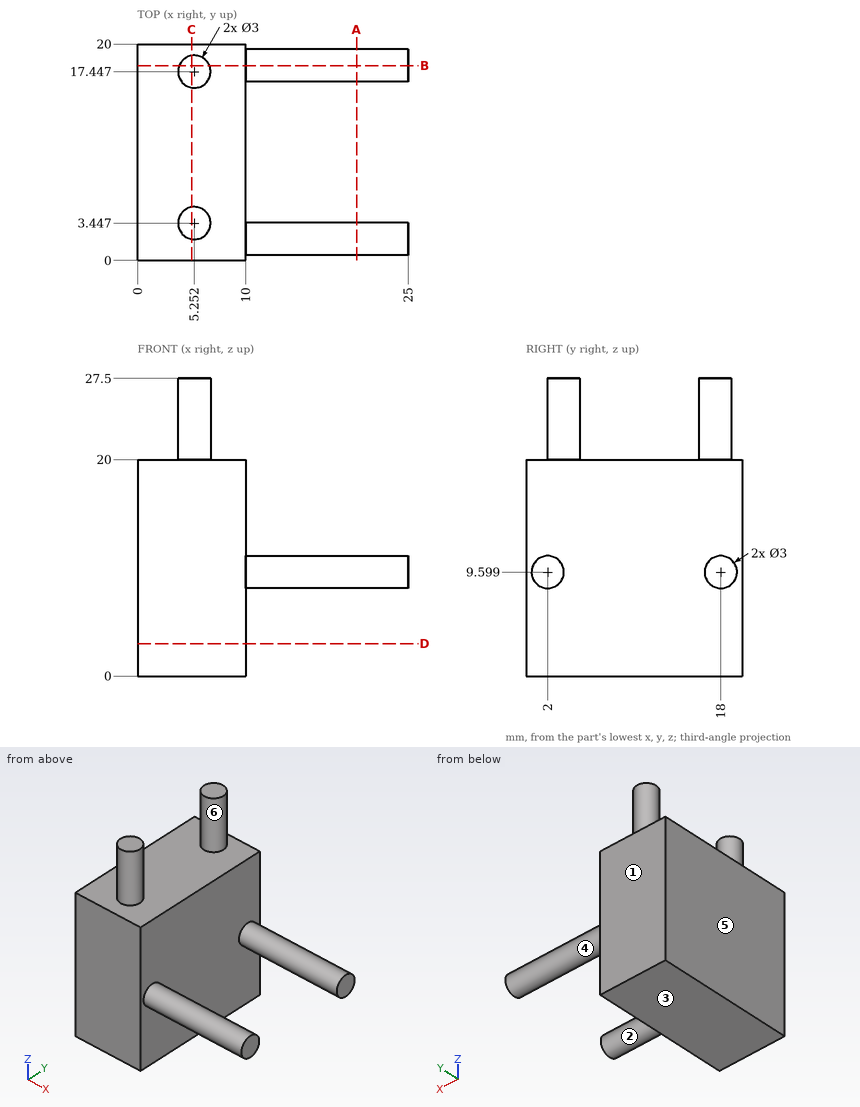
Could you check a few things on this drawing? It's one solid part, dimensions in mm from its lowest x, y, z. A direction names the side the tool comes from. Round coordinates to 2 decimals unless told otherwise and drop trailing zeros. Loops run counter-clockwise (first coordinate to the right, second up) from the corner with the lowest first, then second, coordinate; pieces in that order, holes last. Notation, with made-up numbers: (2.5, 67) -> (54.5, 67) arc R18 ccw to (54.5, 82) -> close; hole circle Ø1 at (-21, 48.5). An arc over 180 degrees is marked (long way). One line per item, written item: value. Start each with the question number.
1. If I drill on probe 1 along X at (y, z) = (15.5, 6.75); probe 2 along Z at (x, y) = (9, 9.25); probe 3 along Z at (x, y) = (23, 18), over which ranges is the centre line in solid material (lowest first)?
2. If we section it at D-D, the plane z = 3: Write out the boundary of the cut face in (x, y), then the cut area to 3 significant figures.
3. If we mould it in two halves opening along Y, with no side actions, what happens to the marked faces 1, 2 and 3? For each: pulls with the +Y half, pulls with the -Y half, needs draft (parallel to the pull), parting line crosses it, or undercut.
4. For the marked faces 4, 5 and 6, which set-ups out of +Z, -Z, +X, -X, +Y, -Y let a thin tool reach every point of the face, with its end or its side?
5. If we section it at B-B, the plane y = 18: Write out the boundary of the cut face in (x, z).
6. For pin 1 (2 mm diameter, centred on y = 10, z = 17, fed in from -X); pin 2 (8 mm diameter, centred on x = 2.5, y = 9, fed in from +Z); pin 3 (2 mm diameter, centred on x = 3.5, z = 23, fed in from -Y); pin 4 (1 mm diameter, centred on y = 12, z = 22, fed in from -X), each with a flat end and sliding along its axis, tell me the tip position at first contact or that it passes through.
7. If we section it at A-A, the plane x = 20.25: Write out the boundary of the cut face in (y, z).
8. If we section it at C-C, the plane x = 5: Write out the boundary of the cut face in (y, z), then the cut area to 3 significant figures.
Calculated:
1. probe 1: x = 0 to 10
1. probe 2: z = 0 to 20
1. probe 3: z = 8.1 to 11.1
2. outline: (0, 0) -> (10, 0) -> (10, 20) -> (0, 20) -> close
2. area: 200 mm²
3. face 1: pulls with the +Y half
3. face 2: undercut
3. face 3: needs draft
4. face 4: +X
4. face 5: +Z, -Z, -X, +Y, -Y
4. face 6: +Z
5. outline: (0, 0) -> (10, 0) -> (10, 8.1) -> (25, 8.1) -> (25, 11.1) -> (10, 11.1) -> (10, 20) -> (6.65, 20) -> (6.65, 27.5) -> (3.86, 27.5) -> (3.86, 20) -> (0, 20) -> close
6. pin 1: stops at x = 0
6. pin 2: stops at z = 20
6. pin 3: stops at y = 2.15
6. pin 4: passes through
7. outline: circle Ø3 at (2, 9.6); circle Ø3 at (18, 9.6)
8. outline: (0, 0) -> (20, 0) -> (20, 20) -> (18.93, 20) -> (18.93, 27.5) -> (15.97, 27.5) -> (15.97, 20) -> (4.93, 20) -> (4.93, 27.5) -> (1.97, 27.5) -> (1.97, 20) -> (0, 20) -> close
8. area: 444 mm²
